Verification items for the finished model (mm, model axes). A direction names the side the tool comes from. Round coordinates to 2 decimals unless told otherwise and drop trailing zeros. Order: outer loops, then holes, each group sorted by start corner. A loop starts at its lowest first (then second) coordinate and runs counter-clockwise, first axis right, second up.
```python
from build123d import *

# Parameters (mm, degrees)
EXTRUDE_1_DEPTH     = 6
SKETCH_2_R          = 5.5
EXTRUDE_2_DEPTH     = 6
FILLET_1_R          = 3
CUT_EXTRUDE_1_DEPTH = 99.325146161


with BuildPart() as part:
    # Эскиз1 → Бобышка-Вытянуть1 (new body)
    with BuildSketch(Plane.XY):
        with BuildLine():
            Line((-60, 0), (-60, 23.629297392))
            ThreePointArc((-60, 23.629297392), (-58.433914458, 29.002293475), (-54.226182617, 32.692375262))
            Line((-54.226182617, 32.692375262), (14.434543456, 64.709397645))
            ThreePointArc((14.434543456, 64.709397645), (25, 67.051702969), (35.565456544, 64.709397645))
            Line((35.565456544, 64.709397645), (54.226182617, 56.00775817))
            ThreePointArc((54.226182617, 56.00775817), (58.433914458, 52.317676383), (60, 46.9446803))
            Line((60, 46.9446803), (60, 0))
            Line((60, 0), (-60, 0))
        make_face()
    extrude(amount=EXTRUDE_1_DEPTH)

    # Эскиз2 → Бобышка-Вытянуть2 (add)
    with BuildSketch(Plane.XZ):
        with BuildLine():
            Line((-60, 6), (60, 6))
            Line((60, 6), (60, 22.249778574))
            ThreePointArc((60, 22.249778574), (57.933533403, 28.337392864), (52.588190451, 31.909036837))
            Line((52.588190451, 31.909036837), (2.588190451, 45.306496459))
            ThreePointArc((2.588190451, 45.306496459), (0, 45.647238196), (-2.588190451, 45.306496459))
            Line((-2.588190451, 45.306496459), (-52.588190451, 31.909036837))
            ThreePointArc((-52.588190451, 31.909036837), (-57.933533403, 28.337392864), (-60, 22.249778574))
            Line((-60, 22.249778574), (-60, 6))
        make_face()
        with Locations(Location((-50, 22.249778574, 0), (0, 0, 270))):
            Circle(SKETCH_2_R, mode=Mode.SUBTRACT)
        with Locations(Location((0, 35.647238196, 0), (0, 0, 270))):
            Circle(SKETCH_2_R, mode=Mode.SUBTRACT)
        with Locations(Location((50, 22.249778574, 0), (0, 0, 270))):
            Circle(SKETCH_2_R, mode=Mode.SUBTRACT)
    extrude(amount=-EXTRUDE_2_DEPTH)

    # Скругление1
    fillet_1_edges = [part.edges().sort_by_distance(p)[0] for p in [
        (0, 6, 6),
    ]]
    fillet(fillet_1_edges, radius=FILLET_1_R)

    # Эскиз3 → Вырез-Вытянуть1 (cut, through all)
    with BuildSketch(Plane.XY.offset(6)):
        with BuildLine():
            Line((51.267854785, 49.663603661), (32.607128711, 58.365243136))
            ThreePointArc((32.607128711, 58.365243136), (25, 60.051702969), (17.392871289, 58.365243136))
            Line((17.392871289, 58.365243136), (-51.267854785, 26.348220753))
            ThreePointArc((-51.267854785, 26.348220753), (-52.718923361, 22.361442607), (-48.732145215, 20.910374031))
            Line((-48.732145215, 20.910374031), (19.928580859, 52.927396414))
            ThreePointArc((19.928580859, 52.927396414), (25, 54.051702969), (30.071419141, 52.927396414))
            Line((30.071419141, 52.927396414), (48.732145215, 44.225756939))
            ThreePointArc((48.732145215, 44.225756939), (52.718923361, 45.676825514), (51.267854785, 49.663603661))
        make_face()
    extrude(amount=-CUT_EXTRUDE_1_DEPTH, mode=Mode.SUBTRACT)


solid = part.part
```
1) Draft check along Z on faces 1 (the cylindrical face through (0.037, 2.958, 45.647)), 2 (the flat face through (-16.46, 42.58, 3.04)), 3 (the cylindrical face through (1.65, 2.96, 30.4)). Enter one of: released by +Z, released by -Z, zero draft, split by the parting line, or undercut.
2) Go/stop test with flat-tipped pins: pin 1 Ø5 at (x, y) = (25, 59) entering from +Z; pin 2 Ø6.5 at (x, z) = (50, 22.25) entering from +Y (1 decimal). Record where each tip stops, or that it passes through.
3) Sectioned sample at B-B on x = -11.5. Record the cut outline in (y, z), then the cut area to 3 significant figures.
4) Sectioned sample at A-A on y = 31. Record the cut outline in (x, z), then the cut area to 3 significant figures.
5) Sectioned sample at C-C on z = 4. Record the cut outline in (x, y), then the cut area to 3 significant figures.
6) Tool access check on faces 4 (the flat face through (-14.882, 36.695, 3.042)), 5 (the flat face through (27.938, 2.958, 38.514)), 6 (the flat face through (-1, 6, 24)). Record the directions out of +Z, -Z, +X, -X, +Y, -Y that give a thin tool (end or side, any length) a straight path to the whole face; none if there is none.
7) Scan lines: probe 1 along X at (y, z) = (3, 26); probe 2 along Y at (x, z) = (-34, 26.5). Record each from-to range of solid material in increasing order.
8) Sectioned sample at D-D on x = -50. Record the cut outline in (y, z).
Returned:
1. face 1: released by +Z
1. face 2: zero draft
1. face 3: undercut
2. pin 1: stops at z = 6
2. pin 2: passes through
3. outline: (0, 0) - (38.27, 0) - (38.27, 6) - (9, 6) arc R3 cw to (6, 9) - (6, 42.92) - (0, 42.92) - close; (44.89, 0) - (52.62, 0) - (52.62, 6) - (44.89, 6) - close
3. area: 499 mm2
4. outline: (-56.76, 0) - (-41.29, 0) - (-41.29, 6) - (-56.76, 6) - close; (-27.09, 0) - (60, 0) - (60, 6) - (-27.09, 6) - close
4. area: 615 mm2
5. outline: (-60, 0) - (60, 0) - (60, 46.94) arc R10 ccw to (54.23, 56.01) - (35.57, 64.71) arc R25 ccw to (14.43, 64.71) - (-54.23, 32.69) arc R10 ccw to (-60, 23.63) - close; hole (-51.27, 26.35) arc R3 ccw to (-48.73, 20.91) - (19.93, 52.93) arc R12 cw to (30.07, 52.93) - (48.73, 44.23) arc R3 ccw to (51.27, 49.66) - (32.61, 58.37) arc R18 ccw to (17.39, 58.37) - close
5. area: 5,670 mm2
6. face 4: +Z, -Z
6. face 5: +Z, +X, +Y, -Y
6. face 6: +Z, +X, -X, +Y
7. probe 1: x = -59.27 to -54.02, -45.98 to 45.98, 54.02 to 59.27
7. probe 2: y = 0 to 6
8. outline: (0, 0) - (20.63, 0) - (20.63, 6) - (9, 6) arc R3 cw to (6, 9) - (6, 16.75) - (0, 16.75) - close; (0, 27.75) - (6, 27.75) - (6, 32.6) - (0, 32.6) - close; (26.94, 0) - (34.66, 0) - (34.66, 6) - (26.94, 6) - close
